```python
from build123d import *

# Parameters (mm, degrees)
F1_DEPTH = 7.9375
F3_DEPTH = 7.9385
F4_SIZE  = 0.635


with BuildPart() as f1:
    # F0 (on Front) → F1 (new body)
    with BuildSketch(Plane.XZ):
        with BuildLine():
            Line((0, 7.9375), (0, 0))
            ThreePointArc((0, 0), (50.8, -3.3566973387), (101.6, 0))
            Line((101.6, 0), (101.6, 7.9375))
            ThreePointArc((101.6, 7.9375), (50.8, 11.2941973387), (0, 7.9375))
        make_face()
    extrude(amount=F1_DEPTH)

    # F2 (on face) → F3 (cut, through all)
    with BuildSketch(Plane.XZ.offset(7.9375)):
        with BuildLine():
            Line((48.9026334039, 2.11875), (52.6973665961, 2.11875))
            ThreePointArc((52.6973665961, 2.11875), (50.8, 6.61875), (48.9026334039, 2.11875))
        make_face()
    extrude(amount=-F3_DEPTH, mode=Mode.SUBTRACT)

    # F4
    f4_edges = [f1.edges().sort_by_distance(p)[0] for p in [
        (50.8, -7.9375, 11.294197),
        (101.6, -7.9375, 3.96875),
        (0, -7.9375, 3.96875),
        (50.8, -7.9375, -3.356697),
        (50.8, -7.9375, 2.11875),
        (50.8, -7.9375, 6.61875),
        (50.8, 0, 11.294197),
        (101.6, 0, 3.96875),
        (0, 0, 3.96875),
        (50.8, 0, -3.356697),
        (50.8, 0, 2.11875),
        (50.8, 0, 6.61875),
    ]]
    chamfer(f4_edges, length=F4_SIZE)


solid = f1.part
```
Geometry check sheet. Reference: the model listing, model coordinates, mm. Round coordinates to 2 decimals unless told otherwise and drop trailing zeros. Loops run counter-clockwise (first coordinate to the right, second up) from the corner with the lowest first, then second, coordinate; pieces in that order, holes last. Notation, with made-up numbers: (-13.5, -35) - (30.5, -35) arc R20 cw to (30.5, -17) - close; hole circle Ø4 at (-14.75, 64.5). An arc over 180 degrees is marked (long way). Write each question's results on one line, items separated by ' | '. Start each with the question number.
Q1. Cross-section at A-A on x = 50.8. Enter the section's corners in (y, z) (1 decimal), and give its area (3 significant figures).
Q2. Release check for a two-part mould opening along Z. For faces 1 (the cylindrical face through (51.513, -3.922, 11.294)), 2 (the conical face through (50.09, -7.77, -2.89)), 3 (the flat face through (51, -4, 2.119)) record: +Z half, -Z half, draft (parallel to the pull), parting line (faces both ways), or undercut.
Q3. Gauge pin test, flat end, axial feed: P1, Ø1.9, axis at x = 50.5, y = -5, coming from the +Z side. Record the tip position at first contact, or that the pin passes through.
Q4. Thickness scan on line 1 (Z direction, x = 50.8, y = -4.75); line 2 (X direction, y = -4, z = 4); line 3 (Z direction, x = 54, y = -2.5). Record the ranges inside material, lowest first. Write a range as [from, to].
Q5. Cross-section at B-B on y = -3.75. Enter the section's corners in (x, z).
Answers below:
1) outline: (-7.9, -2.7) - (-7.3, -3.4) - (-0.6, -3.4) - (0, -2.7) - (0, 1.5) - (-0.6, 2.1) - (-7.3, 2.1) - (-7.9, 1.5) - close; (-7.9, 7.3) - (-7.3, 6.6) - (-0.6, 6.6) - (0, 7.3) - (0, 10.7) - (-0.6, 11.3) - (-7.3, 11.3) - (-7.9, 10.7) - close | area: 79.0 mm²
2) face 1: +Z half | face 2: -Z half | face 3: undercut
3) P1: stops at z = 11.29
4) line 1: z = [-3.36, 2.12], [6.62, 11.29] | line 2: x = [0, 48.15], [53.45, 101.6] | line 3: z = [-3.34, 11.28]
5) outline: (0, 0) arc R386.08 ccw to (101.6, 0) - (101.6, 7.94) arc R386.08 ccw to (0, 7.94) - close; hole (48.9, 2.12) - (52.7, 2.12) arc R2.65 ccw (long way) to start
